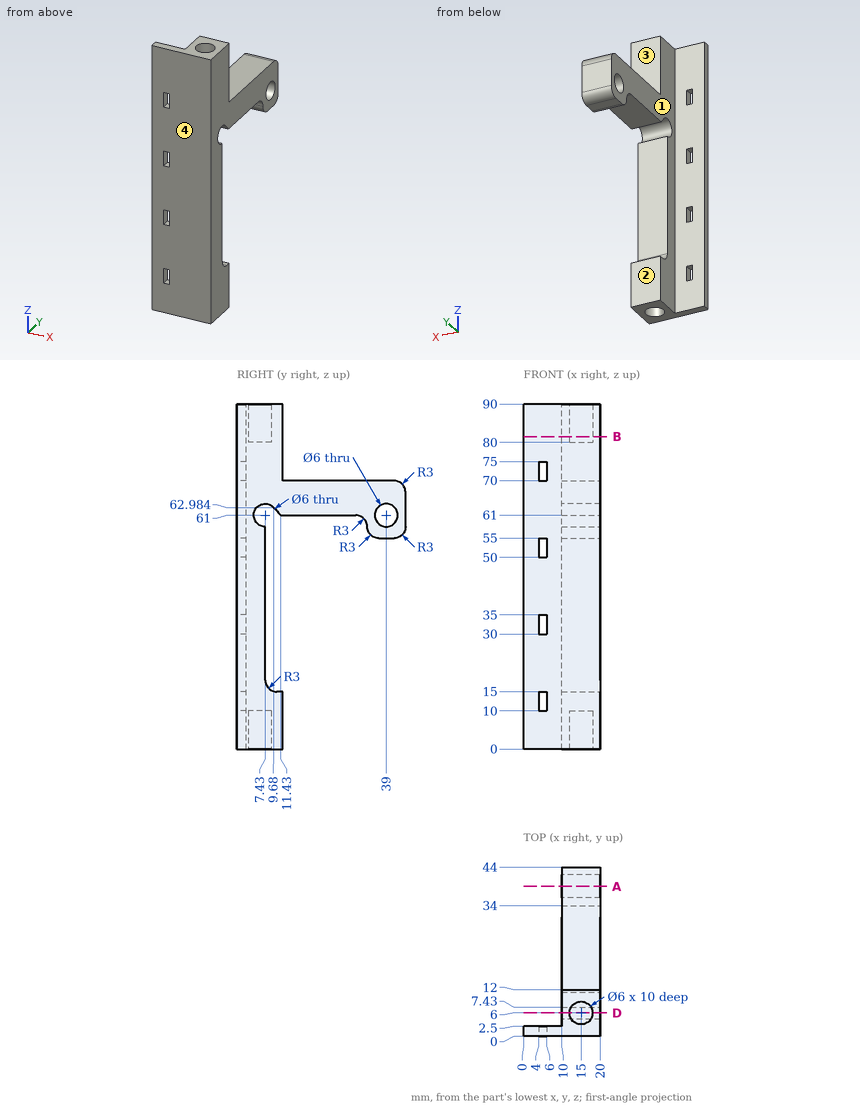
Part print with two shaded views. Sizes in mm from the minimum x, y, z corner. A direction names the side the tool comes from. Give positions to 0.01 mm unless a question says otherwise; leave off trailing zeros. Order: outer loops, then holes, each group sorted by start corner. A loop starts at its lowest first (then second) coordinate and runs counter-clockwise, first axis right, second up. Notation, with made-up numbers: M -17.5,-0.5 L 19.5,-0.5 A20 ccw 19.5,31.5 Z; hole C -10,59 d3. An arc over 180 degrees is marked long. Write item = value, one per line.
Q1. Drill centre lines: line 1 (Y direction, x = 15, z = 83); line 2 (Y direction, x = 8.5, z = 40); line 3 (X direction, y = 23, z = 64). Where is each one in solid material? Low to high. Write a range as [from, to].
Derived:
line_1 = [0, 3], [9, 12]
line_2 = [0, 2.5]
line_3 = [10, 20]
Q2. Flat gauge pins, fed straight in: pin 1 (8 mm diameter, centred on x = 17, y = 22.5, fed in from +Z); pin 2 (3 mm diameter, centred on x = 12.5, z = 10.5, fed in from +Y); pin 3 (1 mm diameter, centred on x = 7, z = 40, fed in from +Y); pin 4 (3 mm diameter, centred on x = 8, y = 24, fed in from -Z). Where does each tip first touch, or does it go through?
Derived:
pin_1 = 70
pin_2 = 12
pin_3 = 2.5
pin_4 = through
Q3. Cut at D-D, the plane y = 6. List the corners of the cut face in (x, z), then the cut area to 3 significant figures.
Derived:
outline = M 10,0 L 12,0 L 12,10 L 18,10 L 18,0 L 20,0 L 20,58.36 L 10,58.36 Z; M 10,63.64 L 20,63.64 L 20,90 L 18,90 L 18,80 L 12,80 L 12,90 L 10,90 Z
area = 727 mm2
Q4. Cut at A-A, the plane y = 39. List the corners of the cut face in (x, z).
Derived:
outline = M 10,55 L 20,55 L 20,58 L 10,58 Z; M 10,64 L 20,64 L 20,70 L 10,70 Z
Q5. Tool access for the marked faces 1, 2, 3 and 4: list every direction of +Z, -Z, +X, -X, +Y, -Y with a clear straight run to the whole face (end or side of a thin tool).
Derived:
face_1 = +Z, -Z, -X, +Y
face_2 = -Z, +X, -X, +Y
face_3 = +Z, +X, -X, +Y
face_4 = +Z, -Z, +X, -X, -Y
Q6. Cut at B-B, the plane z = 81.5. List the corners of the cut face in (x, y).
Derived:
outline = M 0,0 L 20,0 L 20,12 L 10,12 L 10,2.5 L 0,2.5 Z; hole C 15,6 d6
